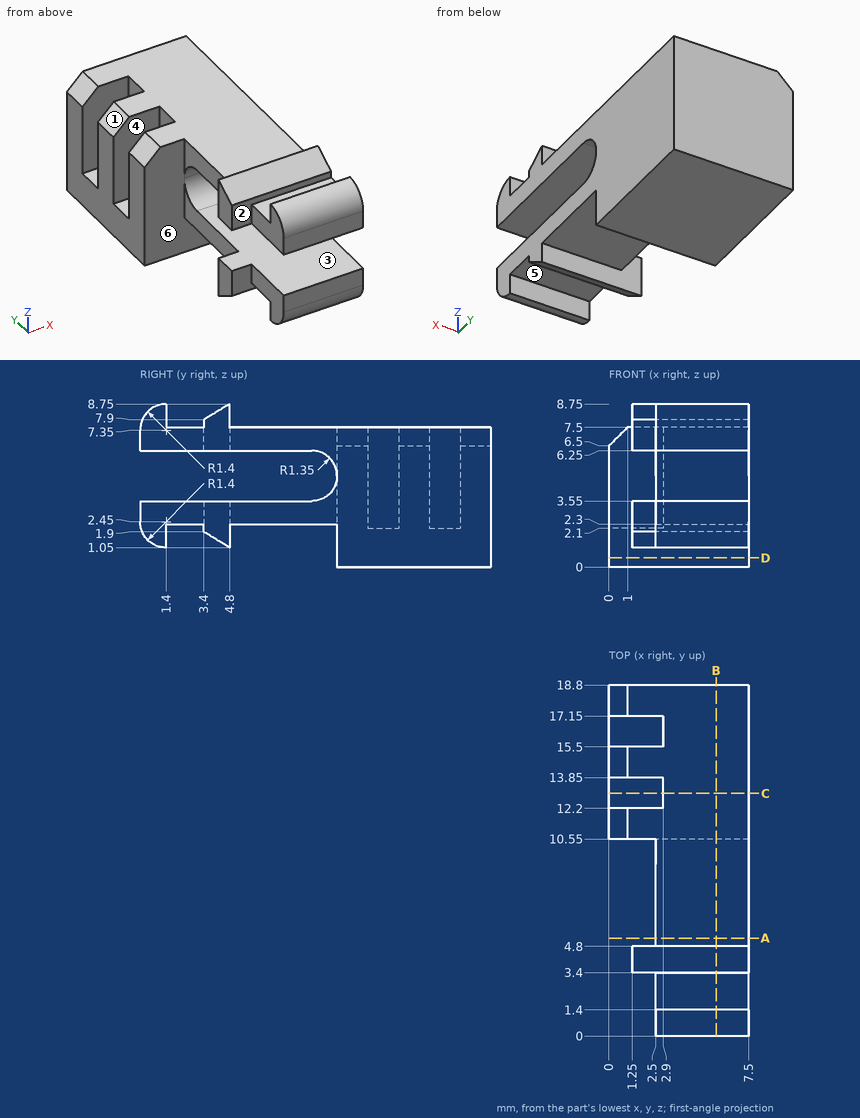
Answer from the drawing. Dimensions are ordinates in mm from the lowest x, y and z of the part. A direction names the side the tool comes from. Coordinates: 2 decimals unless noted, no trailing zeros. Write each loop counter-clockwise with the first axis right and the second up, starting at its lowest first coordinate (ties: lowest second). Pieces come first, ordered by that corner, then holes. Notation, with made-up numbers: M -36.75,74 L -26.75,74 A16 ccw -26.75,96 Z; hole C 55,8 d11. An arc over 180 degrees is marked long. Use one line per item in the form item = value. Start each with the question number.
1. A tool of negligible diameter and unlimited length cuts with its end or side. For the marked faces 4, 5 and 6, from which of +Z, -Z, +X, -X, +Y, -Y can it reach the whole face along a straight path? Write none if from no direction.
2. Straight lines are drawn through the part: probe 1 along Y at (x, z) = (2.25, 7.25); probe 2 along Y at (x, z) = (0.5, 3); probe 3 along Z at (x, y) = (7.25, 8.75). For each, find the intervals that lie inside material, in ascending order. Write a range as from..to.
3. The mould has two halves that part along Z. Classify the marked faces 1, 2 and 3: released by +Z, released by -Z, zero draft, split by the parting line, or undercut.
4. The part is cut by section D-D (z = 0.5). Give the vertices of the cut face in (x, y), plus the area to 3 significant figures.
5. The part is cut by section B-B (x = 5.75). Give the vertices of the cut face in (y, z), plus the area to 3 significant figures.
6. The part is cut by section A-A (y = 5.25). Give the vertices of the cut face in (x, z), plus the area to 3 significant figures.
7. Each of these flat-tipped pins is pushed along its axis until it touches: P1, Ø4, axis at y = 6, z = 8, coming from the +X side; P2, Ø0.8, axis at y = 7.5, z = 6.5, coming from the -X side; P3, Ø3, axis at x = 3.5, y = 6.5, coming from the +Z side; P4, Ø0.7, axis at y = 4.5, z = 2, coming from the -X side. Where does it stop, or does it pass through?
8. The part is cut by section C-C (y = 13). Give the vertices of the cut face in (x, z).
Evaluation:
q1.face_4 = +Z, -X
q1.face_5 = -Z, +X, -X
q1.face_6 = -Z, -X
q2.probe_1 = 3.4..4.8, 10.55..12.2, 13.85..15.5, 17.15..18.8
q2.probe_2 = 10.55..12.2, 13.85..15.5, 17.15..18.8
q2.probe_3 = 2.3..3.55, 6.25..7.5
q3.face_1 = released by +Z
q3.face_2 = zero draft
q3.face_3 = undercut
q4.outline = M 0,10.55 L 7.5,10.55 L 7.5,18.8 L 0,18.8 Z
q4.area = 61.9 mm^2
q5.outline = M 0,2.45 A1.4 ccw 1.4,1.05 L 1.4,2.3 L 3.4,2.3 L 3.4,1.9 L 4.8,1.05 L 4.8,2.3 L 10.55,2.3 L 10.55,0 L 18.8,0 L 18.8,7.5 L 4.8,7.5 L 4.8,8.75 L 3.4,7.9 L 3.4,7.5 L 1.4,7.5 L 1.4,8.75 A1.4 ccw 0,7.35 L 0,6.25 L 9.2,6.25 A1.35 cw 10.55,4.9 A1.35 cw 9.2,3.55 L 0,3.55 Z
q5.area = 94.0 mm^2
q6.outline = M 2.5,2.3 L 7.5,2.3 L 7.5,3.55 L 2.5,3.55 Z; M 2.5,6.25 L 7.5,6.25 L 7.5,7.5 L 2.5,7.5 Z
q6.area = 12.5 mm^2
q7.P1 = 7.5
q7.P2 = 2.5
q7.P3 = 7.5
q7.P4 = 1.25
q8.outline = M 0,0 L 7.5,0 L 7.5,7.5 L 2.9,7.5 L 2.9,2.1 L 0,2.1 Z
